Input: dimensioned drawing with shaded views. Units: mm. Origin: part minimum x, y, z. A direction names the side the tool comes from. Round coordinates to 2 decimals unless told otherwise and drop trailing zeros. Write each loop counter-clockwise with the first axis right and the second up, starting at its lowest first coordinate (ties: lowest second). Pieces come first, ordered by that corner, then holes. Notation, with made-up numbers: (75, 82) -> (96, 82) arc R32 ccw to (96, 113) -> close; hole circle Ø11 at (15.5, 61). An arc over 180 degrees is marked (long way). Return JSON: item names as keys, results as strings. Group by question number.
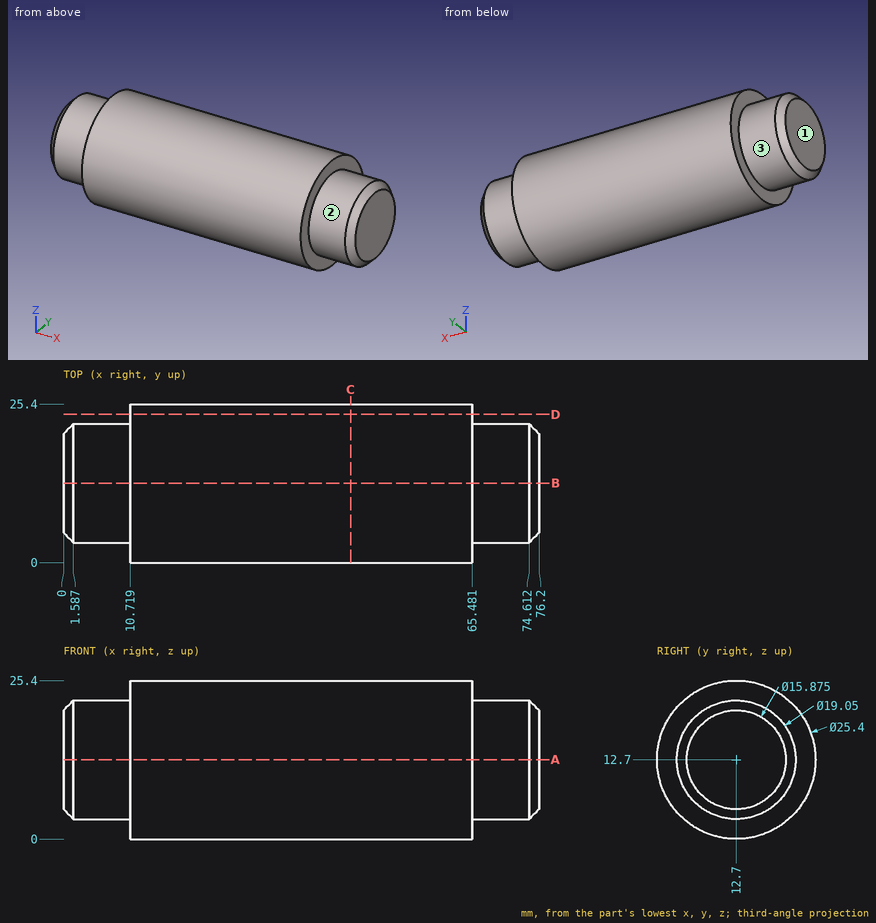
Item 1: Cut plane D-D on y = 23.75. Output: boundary loops of the cut face in (x, z).
Item 2: Cut plane A-A on z = 12.7. Output: boundary loops of the cut face in (x, y) (1 decimal), and give its area (3 significant figures).
Item 3: First-contact query: pin 1 Ø4 at (x, z) = (35, 4.5) entering from +Y (1 decimal); pin 2 Ø1.5 at (y, z) = (5.5, 3) entering from +X; pin 3 Ø6 at (x, z) = (60.5, 8) entering from +Y (1 decimal). Flat tips, straight axial feed; report the tip coordinate or a pass-through.
Item 4: Cut plane C-C on x = 46. Output: boundary loops of the cut face in (y, z), and give its area (3 significant figures).
Item 5: Set-up query: the marked faces 1, 2 and 3. Return all of +Z, -Z, +X, -X, +Y, -Y with unobstructed straight access to the full face (end or side cutting, diameter ignored); none if empty.
Item 6: Material intervals for probe 1 along Y at (x, z) = (60, 13); probe 2 along X at (y, z) = (13.75, 2.25); probe 3 along X at (y, z) = (4, 12.5) (1 decimal), sorted ascending.
Here are the results:
{
 "1": {"outline": "(10.72, 6.44) -> (65.48, 6.44) -> (65.48, 18.96) -> (10.72, 18.96) -> close"},
 "2": {"outline": "(0, 4.8) -> (1.6, 3.2) -> (10.7, 3.2) -> (10.7, 0) -> (65.5, 0) -> (65.5, 3.2) -> (74.6, 3.2) -> (76.2, 4.8) -> (76.2, 20.6) -> (74.6, 22.2) -> (65.5, 22.2) -> (65.5, 25.4) -> (10.7, 25.4) -> (10.7, 22.2) -> (1.6, 22.2) -> (0, 20.6) -> close", "area": "1,790 mm^2"},
 "3": {"pin 1": "stops at y = 23.8", "pin 2": "stops at x = 65.48", "pin 3": "stops at y = 25.3"},
 "4": {"outline": "circle Ø25.4 at (12.7, 12.7)", "area": "507 mm^2"},
 "5": {"face 1": "+Z, -Z, -X, +Y, -Y", "face 2": "+X", "face 3": "-X"},
 "6": {"probe 1": "y = 0 to 25.4", "probe 2": "x = 10.72 to 65.48", "probe 3": "x = 0.8 to 75.4"}
}
